from build123d import *

# Parameters (mm, degrees)
IZIM1_W                          = 40
IZIM1_H                          = 40
Y_KSEKLIK_EKSTR_ZYON1_DEPTH      = 20
KES_EKSTR_ZYON1_DEPTH            = 40
IZIM4_W                          = 10
IZIM4_H                          = 65
Y_KSEKLIK_EKSTR_ZYON2_DEPTH      = 40
KES_EKSTR_ZYON2_DEPTH            = 40
IZIM8_R                          = 15
Y_KSEKLIK_EKSTR_ZYON3_DEPTH      = 5
Y_KSEKLIK_EKSTR_ZYON3_DEPTH_BACK = 30
RADYUS1_R                        = 2
IZIM10_R                         = 15
Y_KSEKLIK_EKSTR_ZYON4_DEPTH      = 10
Y_KSEKLIK_EKSTR_ZYON5_DEPTH      = 10
IZIM18_R                         = 15
Y_KSEKLIK_EKSTR_ZYON6_DEPTH      = 30
IZIM19_R                         = 10
Y_KSEKLIK_EKSTR_ZYON7_DEPTH      = 40
RADYUS2_R                        = 2
RADYUS3_R                        = 2
IZIM21_R                         = 1
KES_EKSTR_ZYON3_DEPTH            = 20
KES_EKSTR_ZYON4_DEPTH            = 20


with BuildPart() as part:
    # izim1 → Y_kseklik-Ekstr_zyon1 (new body, symmetric)
    with BuildSketch(Plane.XY):
        with Locations((-20, 20)):
            Rectangle(IZIM1_W, IZIM1_H)
    extrude(amount=Y_KSEKLIK_EKSTR_ZYON1_DEPTH, both=True)

    # izim3 → Kes-Ekstr_zyon1 (cut)
    with BuildSketch(Plane.XY.offset(20)):
        with BuildLine():
            Line((-40, 40), (-40, 20))
            ThreePointArc((-40, 20), (-34.142135624, 34.142135624), (-20, 40))
            Line((-20, 40), (-40, 40))
        make_face()
        with BuildLine():
            ThreePointArc((-20, 40), (-5.857864376, 34.142135624), (0, 20))
            Line((0, 20), (0, 40))
            Line((0, 40), (-20, 40))
        make_face()
        with BuildLine():
            ThreePointArc((0, 20), (-5.857864376, 5.857864376), (-20, 0))
            Line((-20, 0), (0, 0))
            Line((0, 0), (0, 20))
        make_face()
        with BuildLine():
            Line((-40, 20), (-40, 0))
            Line((-40, 0), (-20, 0))
            ThreePointArc((-20, 0), (-34.142135624, 5.857864376), (-40, 20))
        make_face()
    extrude(amount=-KES_EKSTR_ZYON1_DEPTH, mode=Mode.SUBTRACT)

    # izim4 → Y_kseklik-Ekstr_zyon2 (add)
    with BuildSketch(Plane(origin=(0, 0, 0), x_dir=(0, 0, -1), z_dir=(1, 0, 0))):
        with Locations((15, 52.5)):
            Rectangle(IZIM4_W, IZIM4_H)
    extrude(amount=-Y_KSEKLIK_EKSTR_ZYON2_DEPTH)

    # izim7 → Kes-Ekstr_zyon2 (cut)
    with BuildSketch(Plane.XY.offset(-10)):
        with BuildLine():
            Line((0, 60), (0, 85))
            Line((0, 85), (-40, 85))
            Line((-40, 85), (-40, 60))
            ThreePointArc((-40, 60), (-20, 80), (0, 60))
        make_face()
    extrude(amount=-KES_EKSTR_ZYON2_DEPTH, mode=Mode.SUBTRACT)

    # izim8 → Y_kseklik-Ekstr_zyon3 (add, two sides)
    with BuildSketch(Plane.XY.offset(-10)) as y_kseklik_ekstr_zyon3_sk:
        with Locations((-20, 60)):
            Circle(IZIM8_R)
    extrude(amount=Y_KSEKLIK_EKSTR_ZYON3_DEPTH)
    extrude(y_kseklik_ekstr_zyon3_sk.sketch, amount=-Y_KSEKLIK_EKSTR_ZYON3_DEPTH_BACK)

    # Radyus1
    radyus1_edges = [part.edges().sort_by_distance(p)[0] for p in [
        (-35, 60, -10),
    ]]
    fillet(radyus1_edges, radius=RADYUS1_R)



with BuildPart() as body_2:
    # izim10 → Y_kseklik-Ekstr_zyon4 (new body)
    with BuildSketch(Plane(origin=(0, 0, -40), x_dir=(-1, 0, 0), z_dir=(0, 0, -1))):
        with BuildLine():
            ThreePointArc((45, 60), (20, 85), (-5, 60))
            Line((-5, 60), (-5, 40))
            ThreePointArc((-5, 40), (-6.768788262, 29.424432633), (-11.882623085, 20))
            Line((-11.882623085, 20), (-11.882623085, -18.516208863))
            ThreePointArc((-11.882623085, -18.516208863), (20, -30), (51.882623085, -18.516208863))
            Line((51.882623085, -18.516208863), (51.882623085, 20))
            ThreePointArc((51.882623085, 20), (46.768788262, 29.424432633), (45, 40))
            Line((45, 40), (45, 60))
        make_face()
        with Locations((20, 60)):
            Circle(IZIM10_R, mode=Mode.SUBTRACT)
    extrude(amount=Y_KSEKLIK_EKSTR_ZYON4_DEPTH)


with BuildPart() as part_1:
    add(part.part)

    add(body_2.part)  # Y_kseklik-Ekstr_zyon5 merges body 2
    # izim10_3 → Y_kseklik-Ekstr_zyon5 (add)
    with BuildSketch(Plane(origin=(0, 0, -40), x_dir=(-1, 0, 0), z_dir=(0, 0, -1))):
        with BuildLine():
            ThreePointArc((5, 60), (20, 45), (35, 60))
            Line((35, 60), (5, 60))
        make_face()
        with BuildLine():
            Line((5, 60), (35, 60))
            ThreePointArc((35, 60), (20, 75), (5, 60))
        make_face()
    extrude(amount=Y_KSEKLIK_EKSTR_ZYON5_DEPTH)

    # izim18 → Y_kseklik-Ekstr_zyon6 (add)
    with BuildSketch(Plane(origin=(0, 0, -50), x_dir=(-1, 0, 0), z_dir=(0, 0, -1))):
        with Locations((20, 20)):
            Circle(IZIM18_R)
    extrude(amount=Y_KSEKLIK_EKSTR_ZYON6_DEPTH)

    # izim19 → Y_kseklik-Ekstr_zyon7 (add)
    with BuildSketch(Plane(origin=(0, 0, -80), x_dir=(-1, 0, 0), z_dir=(0, 0, -1))):
        with Locations((20, 20)):
            Circle(IZIM19_R)
    extrude(amount=Y_KSEKLIK_EKSTR_ZYON7_DEPTH)

    # Radyus2
    radyus2_edges = [part_1.edges().sort_by_distance(p)[0] for p in [
        (-5, 20, -50),
    ]]
    fillet(radyus2_edges, radius=RADYUS2_R)

    # Radyus3
    radyus3_edges = [part_1.edges().sort_by_distance(p)[0] for p in [
        (-10, 20, -80),
    ]]
    fillet(radyus3_edges, radius=RADYUS3_R)

    # izim21 → Kes-Ekstr_zyon3 (cut)
    with BuildSketch(Plane(origin=(0, 0, -120), x_dir=(-1, 0, 0), z_dir=(0, 0, -1))):
        with Locations((20, 20)):
            Circle(IZIM21_R)
    extrude(amount=-KES_EKSTR_ZYON3_DEPTH, mode=Mode.SUBTRACT)

    # izim22 → Kes-Ekstr_zyon4 (cut)
    with BuildSketch(Plane(origin=(0, 0, -120), x_dir=(-1, 0, 0), z_dir=(0, 0, -1))):
        with BuildLine():
            Line((17, 27), (20, 27))
            Line((20, 27), (23, 27))
            Line((23, 27), (23, 29.539392014))
            ThreePointArc((23, 29.539392014), (20, 30), (17, 29.539392014))
            Line((17, 29.539392014), (17, 27))
        make_face()
    extrude(amount=-KES_EKSTR_ZYON4_DEPTH, mode=Mode.SUBTRACT)


solid = part_1.part
Here's how the part is built. I have some questions about the finished solid (model axes, mm). A direction names the side the tool comes from. Coordinates: 2 decimals unless noted, no trailing zeros. Order: outer loops, then holes, each group sorted by start corner. A loop starts at its lowest first (then second) coordinate and runs counter-clockwise, first axis right, second up.
Item 1: For faces 1 (the face through (5, 50, -45)), 2 (the face through (-13, 30, -80)), 3 (the face through (-45, 50, -45)), 4 (the face through (-20, 80, -15)), which set-ups out of +Z, -Z, +X, -X, +Y, -Y let a thin tool reach every point of the face, with its end or its side?
Result sheet:
face 1: +Z, -Z, +X, +Y
face 2: -Z
face 3: +Z, -Z, -X, +Y
face 4: +Z, +Y
Item 2: For P1, Ø1.6, axis at x = -19.5, y = 20, coming from the -Z side; P2, Ø3, axis at x = -40.5, y = 24, coming from the -Z side; P3, Ø0.8, axis at y = 28, z = -108.5, coming from the +X side; P4, Ø6.5, axis at x = -20.5, z = -112.5, coming from the +Y side, each with a flat end and sliding along its axis, tell me the tip position at first contact or that it passes through.
Result sheet:
P1: stops at z = -120
P2: stops at z = -50
P3: stops at x = -13.5
P4: stops at y = 29.54
Item 3: If we section it at B-B on z = -26.5: List the corners of the cut face in (x, y) for me.
Result sheet:
outline: circle Ø30 at (-20, 60)
Item 4: If we mould it in two halves opening along X, with no side actions, what happens to faces 5 (the face through (-23.252, 45.357, -6.521)), 6 (the face through (-20, 27, -110)), 7 (the face through (11.883, 1, -45)), 8 (the face through (-20, 29, -100))? For each: +X half, -X half, draft (parallel to the pull), parting line (faces both ways), or undercut.
Result sheet:
face 5: parting line
face 6: undercut
face 7: +X half
face 8: undercut
Item 5: I need wall thicknesses on line 1 (Y direction, x = -20, z = -108.5); line 2 (Z direction, x = 1, y = -17.5); line 3 (Z direction, x = -19.5, y = 6). Which ranges of each line are inside material? Lowest first, please.
Result sheet:
line 1: y = 10 to 19, 21 to 27
line 2: z = -50 to -40
line 3: z = -80 to -40, -20 to 20
Item 6: If we section it at D-D on z = 0: List the corners of the cut face in (x, y) for me.
Result sheet:
outline: circle Ø40 at (-20, 20)
Item 7: If we section it at A-A on z = -109.5: List the corners of the cut face in (x, y) for me, plus the area to 3 significant figures.
Result sheet:
outline: (-23, 27) - (-23, 29.54) arc R10 ccw (long way) to (-17, 29.54) - (-17, 27) - close; hole circle Ø2 at (-20, 20)
area: 294 mm2
Item 8: If we section it at C-C on x = 8.5: List the corners of the cut face in (y, z) for me, plus the area to 3 significant figures.
Result sheet:
outline: (-21.08, -50) - (25.33, -50) - (25.33, -40) - (-21.08, -40) - close
area: 464 mm2
